Study the drawing (mm; zero at the part's minimum x, y, z) and answer. Coordinates: 2 decimals unless noted, no trailing zeros. Write each loop counter-clockwise with the first axis right and the second up, starting at its lowest first coordinate (ties: lowest second). Pieces come first, ordered by that corner, then holes. Notation, with made-up numbers: M 15.5,43 L 36.5,43 A11 cw 36.5,49 Z; hole C 86.25,52 d1. An arc over 180 degrees is marked long. Answer as CSV lines item,"result". Start each with the question number.
(1) Find the intervals of material crossed by L1, parallel to X at y = 1.15, z = 3.5 (1 decimal); L2, parallel to X at y = 3.45, z = 3.25 (1 decimal); L3, parallel to Z at x = 15, y = 2.55 (1 decimal), in increasing order. Write a range as [from, to].
(2) The mould has two halves that part along Z. Classify the marked faces 1, 2 and 3: released by +Z, released by -Z, zero draft, split by the parting line, or undercut.
(3) A cutting plane is placed at B-B on x = 24.5. Give the vertices of the cut face in (y, z), then the cut area to 3 significant figures.
(4) A cutting plane is placed at A-A on y = 3. Count the separate pieces of the cut face and the enclosed holes in it.
(5) A flat-ended cylindrical pin translates along its axis: P1, Ø2, axis at x = 15.772, z = 4.595, coming from the +Y side. Find the tip coordinate at first contact, or state that the pin passes through.
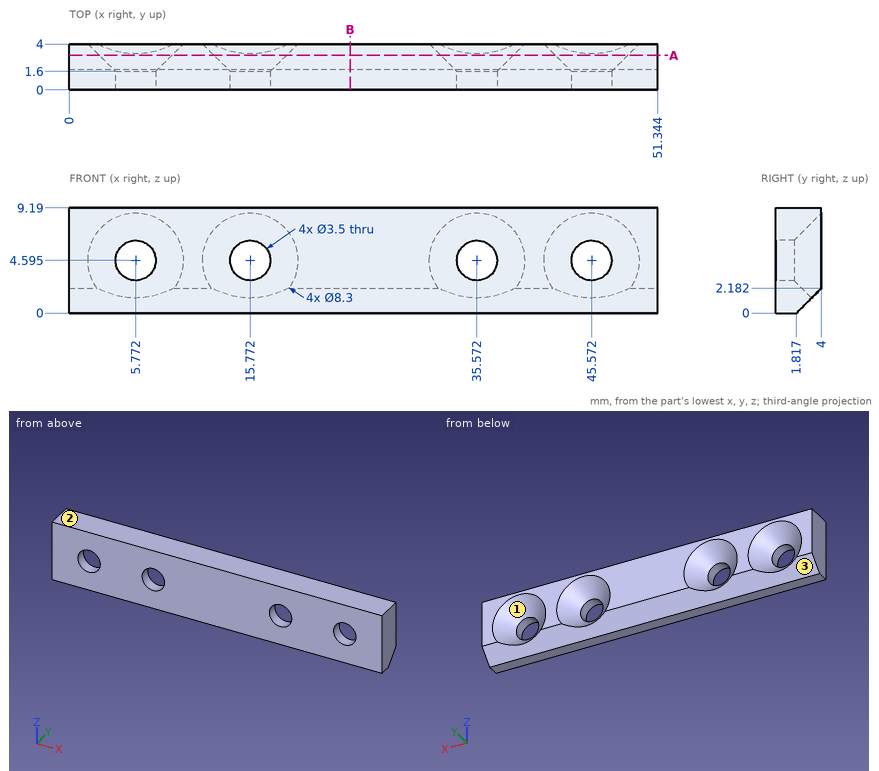
Here are the results:
1,L1,"x = [0, 4.4], [7.1, 14.4], [17.1, 34.2], [36.9, 44.2], [46.9, 51.3]"
1,L2,"x = [0, 2.4], [9.1, 12.4], [19.1, 32.2], [38.9, 42.2], [48.9, 51.3]"
1,L3,"z = [0.7, 2], [7.2, 9.2]"
2,face 1,"undercut"
2,face 2,"released by +Z"
2,face 3,"released by -Z"
3,outline,"M 0,0 L 1.82,0 L 4,2.18 L 4,9.19 L 0,9.19 Z"
3,area,"34.4 mm^2"
4,separate pieces,"1"
4,enclosed holes,"4"
5,P1,"passes through"
